```python
from build123d import *

# Parameters (mm, degrees)
SKETCH_R        = 69.345339
PAD_DEPTH       = 12
SKETCH001_R     = 5
POCKET_DEPTH    = 12.001
SKETCH006_R     = 4
SKETCH006_R_2   = 2.5
POCKET001_DEPTH = 12.001
POCKET002_DEPTH = 405.010966


with BuildPart() as part:
    # Sketch → Pad (new body)
    with BuildSketch(Plane.XY):
        Circle(SKETCH_R)
    extrude(amount=PAD_DEPTH)

    # Sketch001 → Pocket (cut, through all)
    with BuildSketch(Plane(origin=(0, 0, 0), x_dir=(-1, 0, 0), z_dir=(0, 0, -1))):
        Circle(SKETCH001_R)
    extrude(amount=-POCKET_DEPTH, mode=Mode.SUBTRACT)

    # Sketch006 → Pocket001 (cut, through all)
    with BuildSketch(Plane(origin=(0, 0, 0), x_dir=(-1, 0, 0), z_dir=(0, 0, -1))):
        with Locations((0, -26.625)):
            Circle(SKETCH006_R)
        with Locations((-22.5, 16.875)):
            Circle(SKETCH006_R_2)
        with Locations((22.5, 16.875)):
            Circle(SKETCH006_R_2)
    extrude(amount=-POCKET001_DEPTH, mode=Mode.SUBTRACT)

    # Sketch007 → Pocket002 (cut, through all)
    with BuildSketch(Plane.XY.offset(12)):
        with BuildLine():
            Line((7.84131, -14.884662), (16.91337, 4.054655))
            Line((16.91337, 4.054655), (57.3521, -15.315769))
            ThreePointArc((57.3521, -15.315769), (64.614164, -15.137413), (68.738065, -9.157209))
            ThreePointArc((50.968353, -47.021304), (62.776023, -29.460941), (68.738065, -9.157209))
            ThreePointArc((50.968353, -47.021304), (52.945237, -40.089985), (48.54443, -34.381731))
            Line((7.84131, -14.884662), (48.54443, -34.381731))
        make_face()
    pocket002 = extrude(amount=-POCKET002_DEPTH, mode=Mode.SUBTRACT)

    # Mirrored: Pocket002 across Sketch007 V_Axis
    add(pocket002.mirror(Plane(origin=(0, 0, 12), x_dir=(0, 0, 1), z_dir=(1, 0, 0))), mode=Mode.SUBTRACT)


solid = part.part
```
Input: part model. Units: mm. Frame: model coordinates. A direction names the side the tool comes from. Coordinates: 2 decimals unless noted, no trailing zeros. Loops run counter-clockwise (first coordinate to the right, second up) from the corner with the lowest first, then second, coordinate; pieces in that order, holes last. Notation, with made-up numbers: M -5.5,-26 L 43.5,-26 A9 cw 43.5,-17 Z; hole C 35.5,16.25 d3. An arc over 180 degrees is marked long. Answer in a Markdown table with one row per item.
1. Material intervals for line 1 (Y direction, x = 0, z = 6.75) (3 decimals); line 2 (Y direction, x = -4.5, z = 5.75); line 3 (Y direction, x = 22.5, z = 7) (3 decimals), sorted ascending.
Response:
| item | result |
|---|---|
| line 1 | y = -69.345 to -30.625, -22.625 to -5, 5 to 69.345 |
| line 2 | y = -69.2 to -2.18, 2.18 to 69.2 |
| line 3 | y = -65.594 to -21.906, 1.379 to 14.375, 19.375 to 65.594 |
2. Reachability of faces 1 (the flat face through (36.85, -5.495, 6.084)), 2 (the cylindrical face through (-52.964, -40.193, 6.084)) from +Z, -Z, +X, -X, +Y, -Y: full face, straight path, thin tool, end or side. Return the list, or none.
Response:
| item | result |
|---|---|
| face 1 | +Z, -Z |
| face 2 | +Z, -Z, -X |
3. Section D-D, the plane z = 6.75. Output: boundary loops of the cut face in (x, y) (3 decimals).
Response:
| item | result |
|---|---|
| outline | M -68.738,-9.157 A8 ccw -57.352,-15.316 L -16.913,4.055 L -7.841,-14.885 L -48.544,-34.382 A8 ccw -50.968,-47.021 A69.345 ccw 50.968,-47.021 A8 ccw 48.544,-34.382 L 7.841,-14.885 L 16.913,4.055 L 57.352,-15.316 A8 ccw 68.738,-9.157 A69.345 ccw long Z; hole C -22.5,16.875 d5; hole C 0,0 d10; hole C 0,-26.625 d8; hole C 22.5,16.875 d5 |
4. Section C-C, the plane x = -43. Output: boundary loops of the cut face in (y, z), then the cut area to 3 significant figures.
Response:
| item | result |
|---|---|
| outline | M -54.4,0 L -31.73,0 L -31.73,12 L -54.4,12 Z; M -8.44,0 L 54.4,0 L 54.4,12 L -8.44,12 Z |
| area | 1,030 mm2 |
5. First-contact query: pin 1 (6 mm diameter, centred on y = -37.5, z = 2, fed in from -X); pin 2 (2 mm diameter, centred on x = 7, z = 7, fed in from -Y); pin 3 (5 mm diameter, centred on x = 0, y = -26.625, fed in from -Z); pin 4 (1.5 mm diameter, centred on y = -11, z = 7, fed in from +X). Flat tips, straight axial feed; report the tip coordinate or a pass-through.
Response:
| item | result |
|---|---|
| pin 1 | stops at x = -53.01 |
| pin 2 | stops at y = -69.09 |
| pin 3 | passes through |
| pin 4 | stops at x = 68.51 |
6. Draft query along Y for faces 3 (the cylindrical face through (0.52, -22.66, 5.92)), 4 (the flat face through (-1, 16, 12)), 5 (the cylindrical face through (-64.5, -15.2, 6.1)). Return one class per face: pulls with the +Y half, pulls with the -Y half, needs draft (parallel to the pull), parting line crosses it, or undercut.
Response:
| item | result |
|---|---|
| face 3 | undercut |
| face 4 | needs draft |
| face 5 | pulls with the -Y half |
7. Section A-A, the plane x = 0. Output: boundary loops of the cut face in (y, z) (3 decimals).
Response:
| item | result |
|---|---|
| outline | M -69.345,0 L -30.625,0 L -30.625,12 L -69.345,12 Z; M -22.625,0 L -5,0 L -5,12 L -22.625,12 Z; M 5,0 L 69.345,0 L 69.345,12 L 5,12 Z |
8. Section B-B, the plane y = -13. Output: boundary loops of the cut face in (x, z).
Response:
| item | result |
|---|---|
| outline | M -67.13,0 L -52.52,0 L -52.52,12 L -67.13,12 Z; M -8.74,0 L 8.74,0 L 8.74,12 L -8.74,12 Z; M 52.52,0 L 67.13,0 L 67.13,12 L 52.52,12 Z |
